Read the model definition and answer for the solid it produces. Units are mm, in the model's axes. Face numbers are marked on the shaded views. A direction names the side the tool comes from. Coordinates: 2 decimals unless noted, no trailing zeros. Order: outer loops, then holes, each group sorted by start corner. A loop starts at its lowest first (then second) coordinate and runs counter-clockwise, first axis right, second up.
from build123d import *

# Parameters (mm, degrees)
BOSS_EXTRUDE1_DEPTH  = 3
BOSS_EXTRUDE4_DEPTH  = 3
SKETCH11_R           = 13
CUT_EXTRUDE2_DEPTH   = 6.5
BOSS_EXTRUDE5_DEPTH  = 3
CUT_EXTRUDE3_DEPTH   = 24
BOSS_EXTRUDE6_DEPTH  = 3
BOSS_EXTRUDE7_DEPTH  = 6
CUT_EXTRUDE4_DEPTH   = 3
BOSS_EXTRUDE8_DEPTH  = 12
BOSS_EXTRUDE10_DEPTH = 3
BOSS_EXTRUDE11_DEPTH = 3
SKETCH21_W           = 9
SKETCH21_H           = 6
CUT_EXTRUDE5_DEPTH   = 5


with BuildPart() as part:
    # Sketch3 → Boss-Extrude1 (new body)
    with BuildSketch(Plane(origin=(0, 0, 0), x_dir=(1, 0, 0), z_dir=(0, 1, 0))):
        with BuildLine():
            ThreePointArc((-3.439345798, 89.282032024), (-25.956006297, 89.282032024), (-14.697676047, 69.782032024))
            ThreePointArc((-14.697676047, 69.782032024), (-5.505287892, 73.589643868), (-1.697676047, 82.782032024))
            ThreePointArc((-1.697676047, 82.782032024), (-2.140640306, 86.14667961), (-3.439345798, 89.282032024))
        make_face()
        with BuildLine():
            ThreePointArc((-3.439345798, 89.282032024), (-0.67063629, 87.395724301), (1.787544185, 85.119486633))
            ThreePointArc((1.787544185, 85.119486633), (24.283086066, 67.204681754), (51.045533135, 56.680373453))
            ThreePointArc((51.045533135, 56.680373453), (54.245903018, 55.689645548), (57.26384818, 54.23502664))
            ThreePointArc((57.26384818, 54.23502664), (46.005517931, 47.73502664), (46.005517931, 34.73502664))
            ThreePointArc((46.005517931, 34.73502664), (43.236808422, 36.621334362), (40.778627947, 38.89757203))
            ThreePointArc((40.778627947, 38.89757203), (18.283086066, 56.812376909), (-8.479361003, 67.336685211))
            ThreePointArc((-8.479361003, 67.336685211), (-11.679730886, 68.327413115), (-14.697676047, 69.782032024))
            ThreePointArc((-14.697676047, 69.782032024), (-3.439345798, 76.282032024), (-3.439345798, 89.282032024))
        make_face()
        with BuildLine():
            ThreePointArc((57.26384818, 54.23502664), (46.005517931, 47.73502664), (46.005517931, 34.73502664))
            ThreePointArc((46.005517931, 34.73502664), (60.628495766, 28.677990898), (70.26384818, 41.23502664))
            ThreePointArc((70.26384818, 41.23502664), (66.456236335, 50.427414795), (57.26384818, 54.23502664))
        make_face()
    extrude(amount=BOSS_EXTRUDE1_DEPTH)

    # Sketch10 → Boss-Extrude4 (add)
    with BuildSketch(Plane(origin=(0, 3, 0), x_dir=(1, 0, 0), z_dir=(0, 1, 0))):
        with BuildLine():
            ThreePointArc((-4.545374861, 88.183955812), (-24.656968191, 88.532032024), (-14.299728684, 71.288919395))
            ThreePointArc((-14.299728684, 71.288919395), (-11.320648952, 69.799088737), (-8.143608603, 68.798625813))
            ThreePointArc((-8.143608603, 68.798625813), (19.033086066, 58.111415015), (41.876829448, 39.91931244))
            ThreePointArc((41.876829448, 39.91931244), (44.33177593, 37.66814625), (47.111546993, 35.833102851))
            ThreePointArc((47.111546993, 35.833102851), (67.223140323, 35.48502664), (56.865900817, 52.728139268))
            ThreePointArc((56.865900817, 52.728139268), (53.886821084, 54.217969926), (50.709780735, 55.21843285))
            ThreePointArc((50.709780735, 55.21843285), (23.533086066, 65.905643649), (0.689342684, 84.097746224))
            ThreePointArc((0.689342684, 84.097746224), (-1.765603798, 86.348912413), (-4.545374861, 88.183955812))
        make_face()
        with BuildLine():
            ThreePointArc((-5.671220706, 87.085879601), (-23.357930085, 87.782032024), (-13.911689713, 72.812968603))
            ThreePointArc((-13.911689713, 72.812968603), (-10.968716852, 71.276238274), (-7.807856203, 70.260566416))
            ThreePointArc((-7.807856203, 70.260566416), (19.783086066, 59.41045312), (42.975030949, 40.941052849))
            ThreePointArc((42.975030949, 40.941052849), (45.435058904, 38.711503158), (48.237392838, 36.931179062))
            ThreePointArc((48.237392838, 36.931179062), (65.924102218, 36.23502664), (56.477861845, 51.20409006))
            ThreePointArc((56.477861845, 51.20409006), (53.534888984, 52.740820389), (50.374028335, 53.756492247))
            ThreePointArc((50.374028335, 53.756492247), (22.783086066, 64.606605543), (-0.408858816, 83.076005814))
            ThreePointArc((-0.408858816, 83.076005814), (-2.868886772, 85.305555505), (-5.671220706, 87.085879601))
        make_face(mode=Mode.SUBTRACT)
    extrude(amount=BOSS_EXTRUDE4_DEPTH)

    # Sketch11 → Cut-Extrude2 (cut, symmetric)
    with BuildSketch(Plane(origin=(0, 3, 0), x_dir=(1, 0, 0), z_dir=(0, 1, 0))):
        with Locations((-14.697676047, 82.782032024)):
            Circle(SKETCH11_R)
        with Locations((57.26384818, 41.23502664)):
            Circle(SKETCH11_R)
    extrude(amount=CUT_EXTRUDE2_DEPTH, both=True, mode=Mode.SUBTRACT)

    # Sketch12 → Boss-Extrude5 (add)
    with BuildSketch(Plane.XZ):
        Polygon((-4.233574432, -69.812376909), (1.766425568, -80.204681754), (46.799746565, -54.204681754), (40.799746565, -43.812376909), align=None)
        Polygon((2.864501779, -76.106605543), (42.701670353, -53.106605543), (39.701670353, -47.91045312), (-0.135498221, -70.91045312), align=None, mode=Mode.SUBTRACT)
    extrude(amount=BOSS_EXTRUDE5_DEPTH)

    # Sketch13 → Cut-Extrude3 (cut)
    with BuildSketch(Plane.XZ):
        Polygon((39.701670353, -47.91045312), (-0.135498221, -70.91045312), (2.864501779, -76.106605543), (42.701670353, -53.106605543), align=None)
    extrude(amount=-CUT_EXTRUDE3_DEPTH, mode=Mode.SUBTRACT)

    # Sketch14 → Boss-Extrude6 (add)
    with BuildSketch(Plane.XZ.offset(3)):
        Polygon((40.799746565, -43.812376909), (-4.233574432, -69.812376909), (1.766425568, -80.204681754), (46.799746565, -54.204681754), align=None)
    extrude(amount=BOSS_EXTRUDE6_DEPTH)

    # Sketch15 → Boss-Extrude7 (add)
    with BuildSketch(Plane(origin=(0, -3, 0), x_dir=(1, 0, 0), z_dir=(0, 1, 0))):
        Polygon((4.194628798, 68.41045312), (6.792705009, 66.91045312), (9.792705009, 72.106605543), (7.194628798, 73.606605543), align=None)
        Polygon((18.019946345, 67.356605543), (15.019946345, 62.16045312), (17.618022557, 60.66045312), (20.618022557, 65.856605543), align=None)
        Polygon((24.948149576, 63.356605543), (21.948149576, 58.16045312), (24.546225787, 56.66045312), (27.546225787, 61.856605543), align=None)
        Polygon((35.773467123, 57.106605543), (32.773467123, 51.91045312), (35.371543334, 50.41045312), (38.371543334, 55.606605543), align=None)
    extrude(amount=BOSS_EXTRUDE7_DEPTH)

    # Sketch16 → Cut-Extrude4 (cut)
    with BuildSketch(Plane(origin=(0, -3, 0), x_dir=(1, 0, 0), z_dir=(0, 1, 0))):
        Polygon((42.701670353, 53.106605543), (38.371543334, 55.606605543), (35.371543334, 50.41045312), (39.701670353, 47.91045312), align=None)
        Polygon((24.948149576, 63.356605543), (20.618022557, 65.856605543), (17.618022557, 60.66045312), (21.948149576, 58.16045312), align=None)
        Polygon((-0.135498221, 70.91045312), (4.194628798, 68.41045312), (7.194628798, 73.606605543), (2.864501779, 76.106605543), align=None)
    extrude(amount=-CUT_EXTRUDE4_DEPTH, mode=Mode.SUBTRACT)

    # Sketch17 → Boss-Extrude8 (add)
    with BuildSketch(Plane.XZ.offset(6)):
        Polygon((46.799746565, -54.204681754), (40.799746565, -43.812376909), (-4.233574432, -69.812376909), (1.766425568, -80.204681754), align=None)
        Polygon((42.701670353, -53.106605543), (39.701670353, -47.91045312), (-0.135498221, -70.91045312), (2.864501779, -76.106605543), align=None, mode=Mode.SUBTRACT)
    extrude(amount=BOSS_EXTRUDE8_DEPTH)

    # Sketch19 → Boss-Extrude10 (add)
    with BuildSketch(Plane.XZ.offset(18)):
        Polygon((2.315463673, -78.155643649), (44.750708459, -53.655643649), (40.250708459, -45.861415015), (-2.184536327, -70.361415015), (-3.483574432, -71.111415015), (-4.233574432, -69.812376909), (40.799746565, -43.812376909), (46.799746565, -54.204681754), (1.766425568, -80.204681754), (1.016425568, -78.905643649), align=None)
    extrude(amount=BOSS_EXTRUDE10_DEPTH)

    # Sketch20 → Boss-Extrude11 (add)
    with BuildSketch(Plane.XZ.offset(21)):
        Polygon((1.766425568, -80.204681754), (46.799746565, -54.204681754), (40.799746565, -43.812376909), (-4.233574432, -69.812376909), align=None)
        Polygon((42.701670353, -53.106605543), (39.701670353, -47.91045312), (-0.135498221, -70.91045312), (2.864501779, -76.106605543), align=None, mode=Mode.SUBTRACT)
    extrude(amount=BOSS_EXTRUDE11_DEPTH)

    # Sketch21 → Cut-Extrude5 (cut)
    with BuildSketch(Plane(origin=(-33.404826775, 0, -19.286285731), x_dir=(-0.5000000000000008, 0, 0.8660254037844383), z_dir=(-0.8660254037844382, 0, -0.5000000000000007))):
        with Locations((-64.342504686, -15)):
            Rectangle(SKETCH21_W, SKETCH21_H)
    extrude(amount=-CUT_EXTRUDE5_DEPTH, mode=Mode.SUBTRACT)


solid = part.part
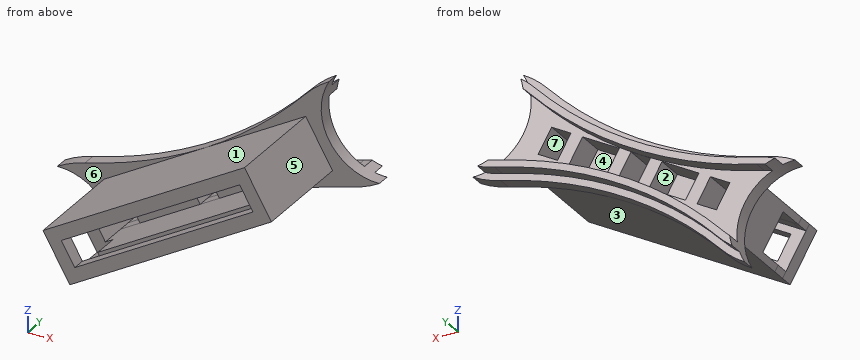
Q1. Straight lines are drawn through the part: L1, parallel to Y at x = 1, z = -76.5; L2, parallel to Y at x = 9, z = -67; L3, parallel to Z at x = 24, y = -15. For each, find the intervals that lie inside material, in ascending order.
Q2. The part is cut by section B-B, the plane y = -11. Determine the outline of the cut face in (x, z).
Q3. Each of these flat-tipped pins is pushed along its axis until it touches: P1, Ø5, axis at x = 1, y = 0.5, coming from the -Z side; P2, Ø10.5, axis at x = 3, z = -55.5, coming from the +Y side; P3, Ø5, axis at y = -5, z = -70, coming from the +X side; P4, Ø1, axis at x = 31, y = -12.5, coming from the -Z side. Where does it stop, or does it pass through?
Q4. The part is cut by section A-A, the plane y = 1.25. Determine the outline of the cut face in (x, z), then the cut area to 3 significant figures.
Q5. Which of the six approach directions +Z, -Z, +X, -X, +Y, -Y give full straight-line access (tool end or side, diameter ignored) to the marked faces 4, 5, 6 and 7?
Q6. Determine the mould class of the marked faces 1, 2 and 3 for opening direction X: +X half, -X half, draft (parallel to the pull), parting line (faces both ways), or undercut.
Computed values:
1. L1: y = -24 to -21, -12 to 3
1. L2: y = -6 to -3
1. L3: z = -67.37 to -63.9, -56.98 to -53.51
2. outline: (-4.23, -69.81) - (1.77, -80.2) - (46.8, -54.2) - (40.8, -43.81) - close; hole (-0.14, -70.91) - (2.86, -76.11) - (42.7, -53.11) - (39.7, -47.91) - close
3. P1: stops at z = -88.03
3. P2: passes through
3. P3: stops at x = 23.77
3. P4: stops at z = -63.62
4. outline: (-14.7, -69.78) arc R13 cw to (-3.44, -89.28) arc R22.52 ccw to (1.79, -85.12) arc R96.91 cw to (51.05, -56.68) arc R22.52 ccw to (57.26, -54.24) arc R13 cw to (46.01, -34.74) arc R22.52 ccw to (40.78, -38.9) arc R96.91 cw to (-8.48, -67.34) arc R22.52 ccw to start; hole (-0.14, -70.91) - (2.86, -76.11) - (7.19, -73.61) - (4.19, -68.41) - close; hole (6.79, -66.91) - (9.79, -72.11) - (18.02, -67.36) - (15.02, -62.16) - close; hole (17.62, -60.66) - (20.62, -65.86) - (24.95, -63.36) - (21.95, -58.16) - close; hole (24.55, -56.66) - (27.55, -61.86) - (35.77, -57.11) - (32.77, -51.91) - close; hole (35.37, -50.41) - (38.37, -55.61) - (42.7, -53.11) - (39.7, -47.91) - close
4. area: 720 mm2
5. face 4: +Y
5. face 5: +Z, +X, -Y
5. face 6: -Y
5. face 7: +Y, -Y
6. face 1: -X half
6. face 2: undercut
6. face 3: +X half
